```python
from build123d import *

# Parameters (mm, degrees)
EXTRUDE_THIN1_DEPTH = 150.8125
FILLET1_R           = 1.016


with BuildPart() as part:
    # Sketch1 → Extrude-Thin1 (new body)
    with BuildSketch(Plane.XY):
        with BuildLine():
            Line((11.90625, 0), (19.84375, 0))
            Line((19.84375, 0), (19.84375, 6.35))
            Line((19.84375, 6.35), (16.611859403, 6.35))
            ThreePointArc((16.611859403, 6.35), (16.819864191, 11.185113028), (14.420873366, 15.388257922))
            ThreePointArc((14.420873366, 15.388257922), (12.164462393, 18.51520612), (11.1125, 22.225))
            Line((11.1125, 22.225), (8.73125, 22.225))
            Line((8.73125, 22.225), (8.73125, 26.9875))
            Line((8.73125, 26.9875), (4.7625, 26.9875))
            Line((4.7625, 26.9875), (4.7625, 11.1125))
            Line((4.7625, 11.1125), (5.7785, 11.1125))
            Line((5.7785, 11.1125), (5.7785, 25.9715))
            Line((5.7785, 25.9715), (7.71525, 25.9715))
            Line((7.71525, 25.9715), (7.71525, 21.209))
            Line((7.71525, 21.209), (10.230316486, 21.209))
            ThreePointArc((10.230316486, 21.209), (11.458524166, 17.661660911), (13.712626283, 14.659806091))
            ThreePointArc((13.712626283, 14.659806091), (15.971237356, 10.225128152), (15.052239099, 5.334))
            Line((15.052239099, 5.334), (18.82775, 5.334))
            Line((18.82775, 5.334), (18.82775, 1.016))
            Line((18.82775, 1.016), (11.90625, 1.016))
            Line((11.90625, 1.016), (11.90625, 0))
        make_face()
    extrude(amount=-EXTRUDE_THIN1_DEPTH)

    # Fillet1
    fillet1_edges = [part.edges().sort_by_distance(p)[0] for p in [
        (4.7625, 26.9875, -75.40625),
        (8.73125, 26.9875, -75.40625),
        (11.1125, 22.225, -75.40625),
        (19.84375, 6.35, -75.40625),
        (19.84375, 0, -75.40625),
        (15.052239099, 5.334, -75.40625),
        (7.71525, 21.209, -75.40625),
    ]]
    fillet(fillet1_edges, radius=FILLET1_R)


solid = part.part
```
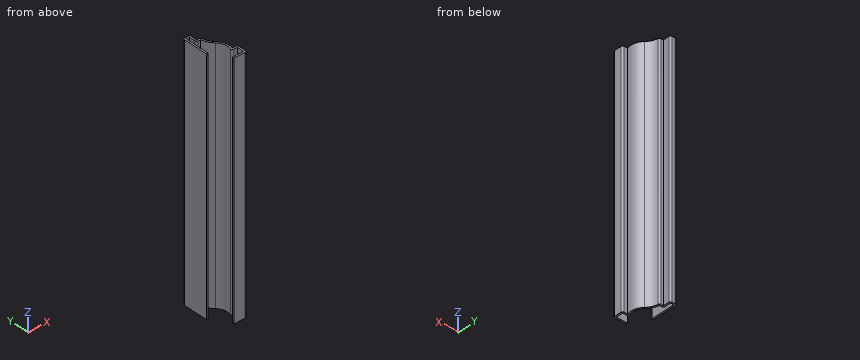
Read the model definition and answer for the solid it produces. Units are mm, in the model's axes. Coordinates: 2 decimals unless noted, no trailing zeros. Order: outer loops, then holes, each group sorted by start corner. A loop starts at its lowest first (then second) coordinate and runs counter-clockwise, first axis right, second up. Notation, with made-up numbers: (77, -5.75) - (136, -5.75) arc R23 cw to (136, 8.25) - close; hole circle Ø2 at (24, -1). An arc over 180 degrees is marked (long way). Answer as a JSON object with one key per item and string values. Group by question number.
Item 1: Consider probe 1 along X at (y, z) = (24.25, -45); probe 2 along Y at (x, z) = (17.75, -122.5); probe 3 along X at (y, z) = (4.75, -37). Determine where each line is inside the solid, lowest interval first. Write a range as from..to.
Item 2: Section D-D (y = 12.5) is taken. Give the vertices of the cut face in (x, z).
Item 3: Section A-A (y = 19.5) is taken. Give the vertices of the cut face in (x, z).
Item 4: Flat-ended cylindrical pins translate along their axes: P1, Ø1.6, axis at x = 10, z = -54, coming from the +Y side (3 decimals); P2, Ø1.3, axis at y = 3.5, z = -90.5, coming from the -X side; P3, Ø4.5, axis at y = 20.5, z = -105.5, coming from the +X side. Find the tip coordinate at first contact, or state that the pin passes through.
Item 5: Section C-C (y = 3) is taken. Give the vertices of the cut face in (x, z).
Results are:
{
 "1": {"probe 1": "x = 4.76..5.78, 7.72..8.73", "probe 2": "y = 0..1.02, 5.33..6.35", "probe 3": "x = 18.83..19.84"},
 "2": {"outline": "(4.76, -150.81) - (5.78, -150.81) - (5.78, 0) - (4.76, 0) - close; (15.27, -150.81) - (16.39, -150.81) - (16.39, 0) - (15.27, 0) - close"},
 "3": {"outline": "(4.76, -150.81) - (5.78, -150.81) - (5.78, 0) - (4.76, 0) - close; (10.67, -150.81) - (11.75, -150.81) - (11.75, 0) - (10.67, 0) - close"},
 "4": {"P1": "stops at y = 22.225", "P2": "stops at x = 18.83", "P3": "stops at x = 12.3"},
 "5": {"outline": "(18.83, -150.81) - (19.84, -150.81) - (19.84, 0) - (18.83, 0) - close"}
}
